Drawing for the job (mm, zero at the part's lowest x, y, z). Give positions to 0.01 mm unless a question says otherwise; leave off trailing zeros. Write each loop counter-clockwise with the first axis right and the second up, starting at its lowest first coordinate (ties: lowest second). Pieces come first, ordered by that corner, then holes. Notation, with made-up numbers: M -13,-18 L 46,-18 A20 cw 46,4 Z; hole C 69,-12.5 d5. An arc over 180 degrees is marked long. Use a Markdown table: item, result. Add a question column.
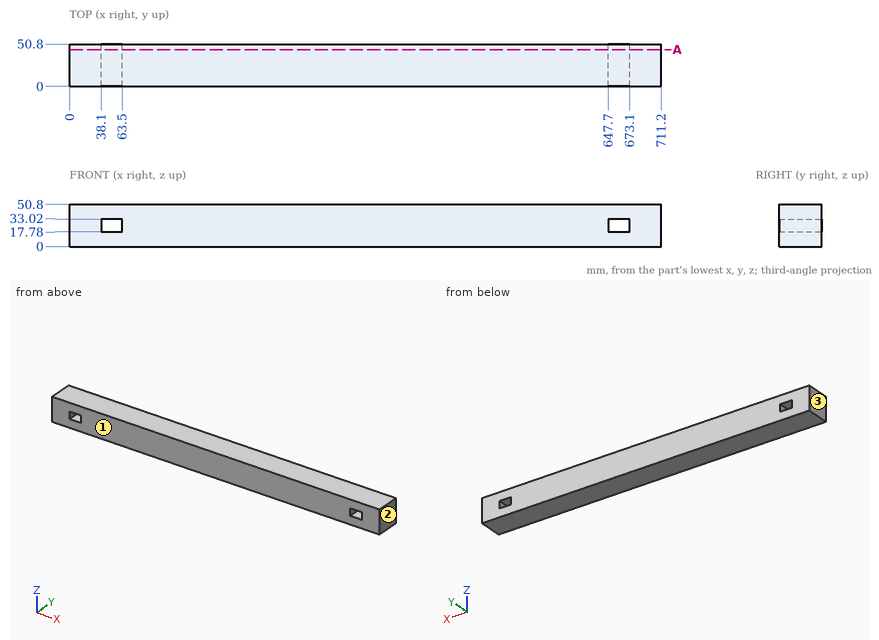
1. Cut at A-A (y = 44). Write the cut outline in (x, z).
2. Drill centre lines: probe 1 along X at (y, z) = (5, 23.5); probe 2 along Z at (x, y) = (652, 9). Where is each one in solid material? Low to high. Write a range as [from, to].
3. Mould opens along X. For the marked faces 1, 2 and 3 say: released by +X, released by -X, zero draft, split by the parting line, or undercut.
4. Flat gauge pin, fed straight in: pin 1 (5 mm diameter, centred on x = 291.5, z = 37, fed in from -Y). Where does the tip first touch, or does it go through?
A:
| question | item | result |
|---|---|---|
| 1 | outline | M 0,0 L 711.2,0 L 711.2,50.8 L 0,50.8 Z; hole M 38.1,17.78 L 63.5,17.78 L 63.5,33.02 L 38.1,33.02 Z; hole M 647.7,17.78 L 673.1,17.78 L 673.1,33.02 L 647.7,33.02 Z |
| 2 | probe 1 | x = [0, 38.1], [63.5, 647.7], [673.1, 711.2] |
| 2 | probe 2 | z = [0, 17.78], [33.02, 50.8] |
| 3 | face 1 | zero draft |
| 3 | face 2 | released by +X |
| 3 | face 3 | released by -X |
| 4 | pin 1 | stops at y = 0 |
